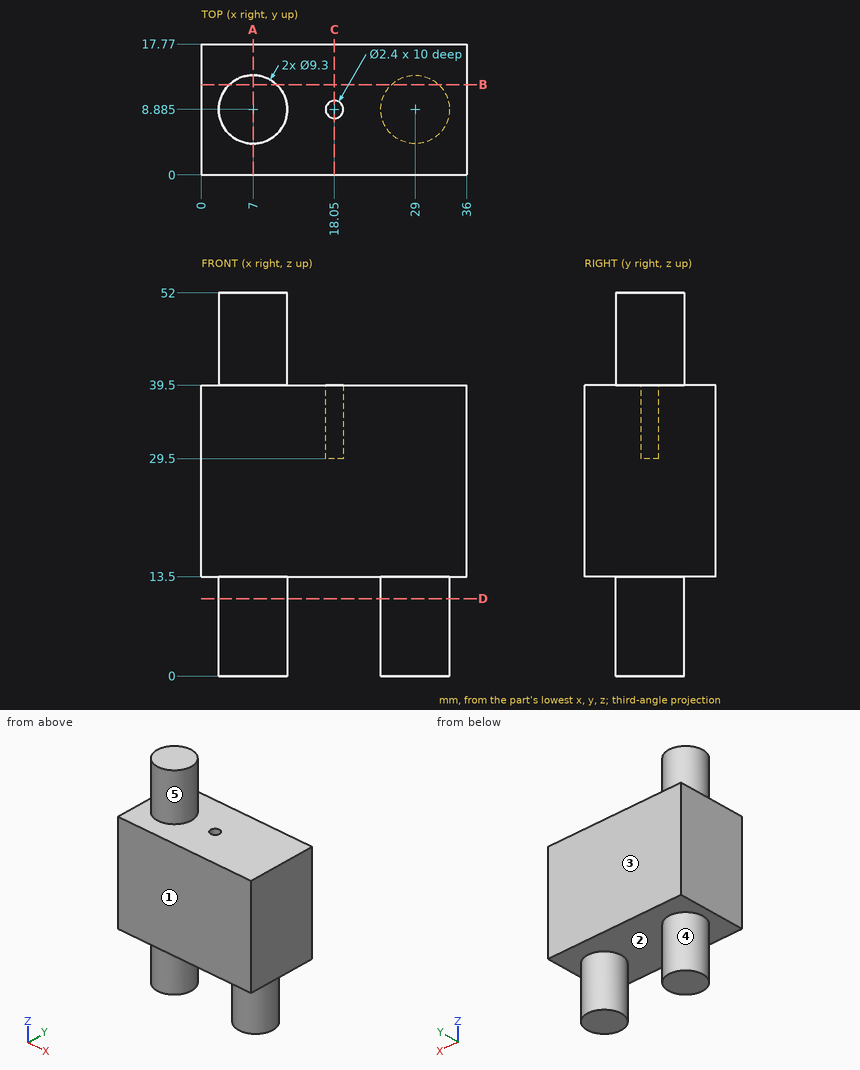
Geometry: see drawing. Coordinates: mm, zero at the bounding-box minimum. A direction names the side the tool comes from. Round coordinates to 2 decimals unless told otherwise and drop trailing zeros. Write each loop counter-clockwise with the first axis right and the second up, starting at its lowest first coordinate (ties: lowest second). Pieces come first, ordered by that corner, then holes. Notation, with made-up numbers: (-39.75, 82.5) - (-13.75, 82.5) arc R23 cw to (-13.75, 121.5) - close; hole circle Ø1 at (-30.75, 32.5). An arc over 180 degrees is marked (long way). Use CSV: the item, a comma, the result in double quotes. Start each with the question number.
(1) Mould query, pull axis X, two halves, no side actions, for the marked faces 3, 4 and 5. Classes: pulls with the +X half, pulls with the -X half, needs draft (parallel to the pull), parting line crosses it, or undercut.
(2) First-contact query: pin 1 Ø1.2 at (x, y) = (18, 8.5) entering from +Z; pin 2 Ø2 at (y, z) = (10, 42.5) entering from +X; pin 3 Ø8 at (x, y) = (25, 12) entering from +Z. Flat tips, straight axial feed; report the tip coordinate or a pass-through.
(3) Cut plane C-C, the plane x = 18.05. Return loops of the section in (y, z) (3 decimals), and give its area (3 significant figures).
(4) Cut plane A-A, the plane x = 7. Return loops of the section in (y, z) (3 decimals).
(5) Material intervals for probe 1 along Y at (x, z) = (18.05, 36.25) (3 decimals); probe 2 along Z at (x, y) = (22, 5.75); probe 3 along Z at (x, y) = (28, 6.25), sorted ascending. Write a range as [from, to].
(6) Cut plane D-D, the plane z = 10.5. Return loops of the section in (x, y) (3 decimals).
(7) Cut plane B-B, the plane y = 12.25. Return loops of the section in (x, z).
(8) Set-up query: the marked faces 1 and 2. Return all of +Z, -Z, +X, -X, +Y, -Y with unobstructed straight access to the full face (end or side cutting, diameter ignored); none if empty.
Geometry says:
1,face 3,"needs draft"
1,face 4,"undercut"
1,face 5,"parting line crosses it"
2,pin 1,"z = 29.5"
2,pin 2,"x = 11.65"
2,pin 3,"z = 39.5"
3,outline,"(0, 13.5) - (17.77, 13.5) - (17.77, 39.5) - (10.085, 39.5) - (10.085, 29.5) - (7.685, 29.5) - (7.685, 39.5) - (0, 39.5) - close"
3,area,"438 mm²"
4,outline,"(0, 13.5) - (4.235, 13.5) - (4.235, 0) - (13.535, 0) - (13.535, 13.5) - (17.77, 13.5) - (17.77, 39.5) - (13.535, 39.5) - (13.535, 52) - (4.235, 52) - (4.235, 39.5) - (0, 39.5) - close"
5,probe 1,"[0, 7.685], [10.085, 17.77]"
5,probe 2,"[13.5, 39.5]"
5,probe 3,"[0, 39.5]"
6,outline,"circle Ø9.3 at (7, 8.885); circle Ø9.3 at (29, 8.885)"
7,outline,"(0, 13.5) - (3.79, 13.5) - (3.79, 0) - (10.21, 0) - (10.21, 13.5) - (25.79, 13.5) - (25.79, 0) - (32.21, 0) - (32.21, 13.5) - (36, 13.5) - (36, 39.5) - (10.21, 39.5) - (10.21, 52) - (3.79, 52) - (3.79, 39.5) - (0, 39.5) - close"
8,face 1,"+Z, -Z, +X, -X, -Y"
8,face 2,"-Z"
